Could you check a few things on this model? Use its own coordinates, in mm. Give positions to 0.01 mm unless a question says otherwise; leave off trailing zeros. Loops run counter-clockwise (first coordinate to the right, second up) from the corner with the lowest first, then second, coordinate; pieces in that order, holes last. Notation, with made-up numbers: (-38.75, 73.25) - (20.25, 73.25) arc R12 cw to (20.25, 96.25) - close; hole circle Ø10 at (35, 7). An arc over 180 degrees is marked (long way). One line per item, written item: value. Start each with the question number.
Q1. I want a section at B-B (z = 3.5). Please give me the cut outline in (x, y).
Q2. I want a section at C-C (x = 73.5). Please give me the cut outline in (y, z), then the cut area to 3 significant figures.
Q3. I'm going to push flat-ended pins straight in: P1, Ø3, axis at x = 72.5, z = -2, coming from the -Y side; P2, Ø3, axis at x = 70.5, z = -2, coming from the +Y side; P3, Ø5, axis at x = 100, z = 0, coming from the -Y side; P4, Ø1, axis at y = 8.5, z = -2, coming from the +X side. Where does each tip first touch, or does it pass through?
Q4. If I drill on line 1 (X direction, y = 6.25, z = 0); line 2 (Z direction, x = 0, y = 8.5); line 3 (X direction, y = 2.75, z = 0), over which ranges is the centre line in solid material (lowest first)? Write a range as from..to.
Q5. I want a section at A-A (y = 11). Please give me the cut outline in (x, z).
Q6. I want a section at D-D (z = -3.75). Please give me the cut outline in (x, y).
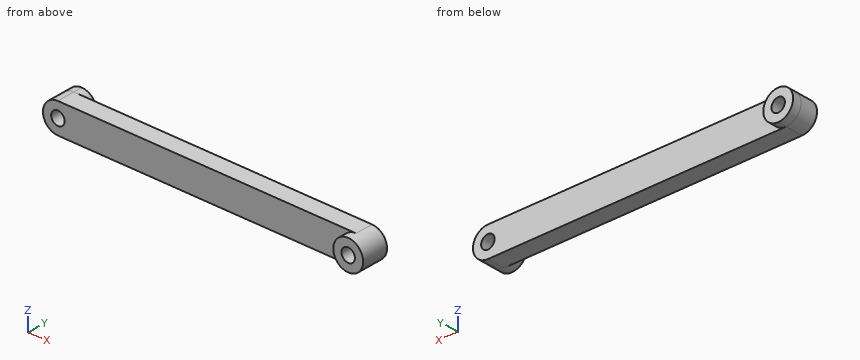
```python
from build123d import *

# Parameters (mm, degrees)
SKETCH1_R               = 2.25
BOSS_EXTRUDE1_DEPTH     = 12
CUT_EXTRUDE_THIN1_START = -3
SKETCH2_R               = 1005
SKETCH2_R_2             = 5
CUT_EXTRUDE_THIN1_DEPTH = 3
SKETCH3_R               = 1005
SKETCH3_R_2             = 5
CUT_EXTRUDE_THIN2_DEPTH = 3


with BuildPart() as part:
    # Sketch1 → Boss-Extrude1 (new body)
    with BuildSketch(Plane(origin=(0, 0, 0), x_dir=(1, 0, 0), z_dir=(0, 1, 0))):
        with BuildLine():
            Line((0, 5), (100, 5))
            ThreePointArc((100, 5), (105, 0), (100, -5))
            Line((100, -5), (0, -5))
            ThreePointArc((0, -5), (-5, 0), (0, 5))
        make_face()
        with Locations(Location((0, 0, 0), (0, 0, 270))):
            Circle(SKETCH1_R, mode=Mode.SUBTRACT)
        with Locations(Location((100, 0, 0), (0, 0, 270))):
            Circle(SKETCH1_R, mode=Mode.SUBTRACT)
    extrude(amount=BOSS_EXTRUDE1_DEPTH)

    # Sketch2 → Cut-Extrude-Thin1 (cut)
    with BuildSketch(Plane(origin=(0, 12, 0), x_dir=(1, 0, 0), z_dir=(0, 1, 0)).offset(CUT_EXTRUDE_THIN1_START)):
        Circle(SKETCH2_R)
        Circle(SKETCH2_R_2, mode=Mode.SUBTRACT)
    extrude(amount=CUT_EXTRUDE_THIN1_DEPTH, mode=Mode.SUBTRACT)

    # Sketch3 → Cut-Extrude-Thin2 (cut)
    with BuildSketch(Plane.XZ):
        with Locations((100, 0)):
            Circle(SKETCH3_R)
        with Locations((100, 0)):
            Circle(SKETCH3_R_2, mode=Mode.SUBTRACT)
    extrude(amount=-CUT_EXTRUDE_THIN2_DEPTH, mode=Mode.SUBTRACT)


solid = part.part
```
Worked answers:
1. outline: (-3.57, 3) - (96.43, 3) - (96.43, 0) - (103.57, 0) - (103.57, 9) - (3.57, 9) - (3.57, 12) - (-3.57, 12) - close
2. outline: (3, -5) - (9, -5) - (9, 5) - (3, 5) - close
2. area: 60.0 mm²
3. P1: stops at y = 3
3. P2: stops at y = 9
3. P3: stops at y = 0
3. P4: stops at x = 104.77
4. line 1: x = -5..-2.25, 2.25..97.75, 102.25..105
4. line 2: z = -5..-2.25, 2.25..5
4. line 3: x = 95..97.75, 102.25..105
5. outline: circle Ø10 at (0, 0); hole circle Ø4.5 at (0, 0)
6. outline: (-3.31, 3) - (96.69, 3) - (96.69, 0) - (103.31, 0) - (103.31, 9) - (3.31, 9) - (3.31, 12) - (-3.31, 12) - close
